Design review of the part shown in the three views and the two pictorial views. Dimensions are in mm from the part's minimum x, y and z. A direction names the side the tool comes from. Give positions to 0.01 mm unless a question says otherwise; leave off trailing zeros. Order: outer loops, then holes, each group sorted by start corner. A loop starts at its lowest first (then second) coordinate and runs counter-clockwise, first axis right, second up.
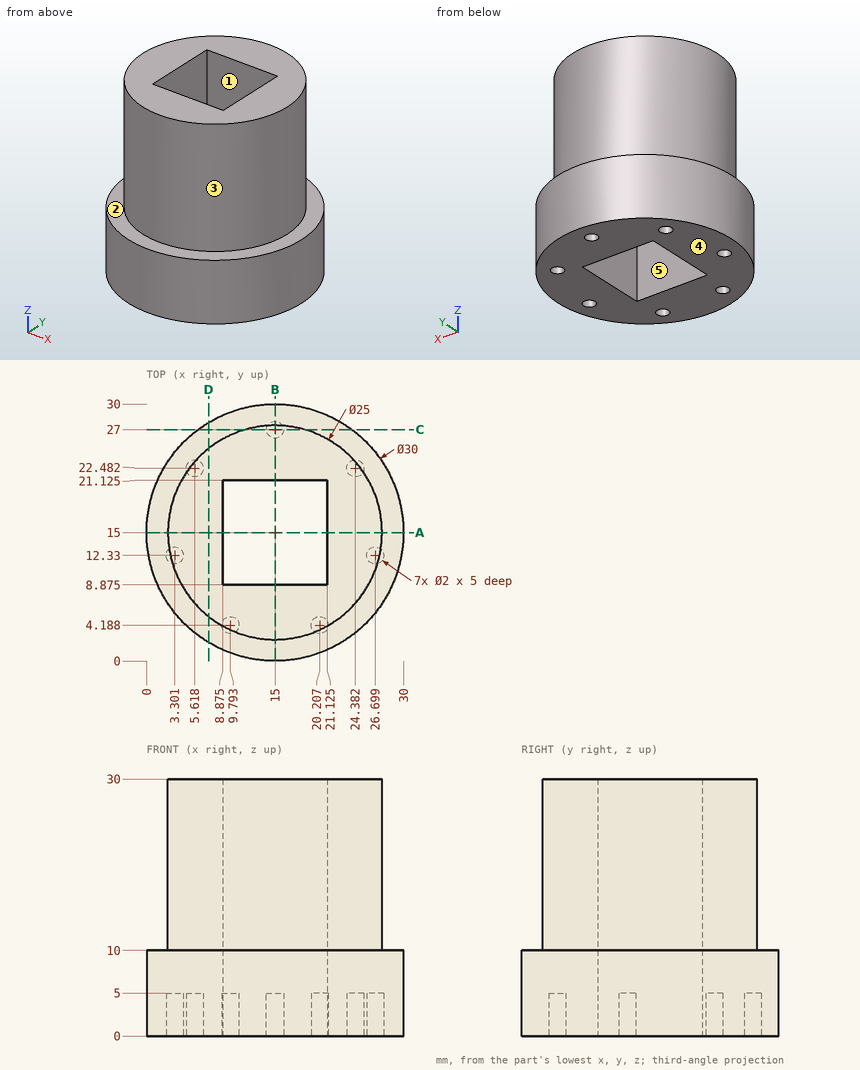
1) Tool access review of the marked faces 4 and 5: name each direction out of +Z, -Z, +X, -X, +Y, -Y from which nothing blocks a thin tool from reaching the whole face with its end or side.
Answer sheet:
face 4: -Z, +X, -X, +Y, -Y
face 5: +Z, -Z
2) Draft analysis for pull direction X (two halves, no side actions). For the marked faces 1, 2 and 3, state which applies: +X half, -X half, draft (parallel to the pull), parting line (faces both ways), or undercut.
Answer sheet:
face 1: undercut
face 2: draft
face 3: parting line
3) We need section B-B on x = 15. Give the boundary of the cut face in (y, z) (1 decimal).
Answer sheet:
outline: (0, 0) - (8.9, 0) - (8.9, 30) - (2.5, 30) - (2.5, 10) - (0, 10) - close; (21.1, 0) - (26, 0) - (26, 5) - (28, 5) - (28, 0) - (30, 0) - (30, 10) - (27.5, 10) - (27.5, 30) - (21.1, 30) - close
4) We need section A-A on y = 15. Give the boundary of the cut face in (x, z) (1 decimal).
Answer sheet:
outline: (0, 0) - (8.9, 0) - (8.9, 30) - (2.5, 30) - (2.5, 10) - (0, 10) - close; (21.1, 0) - (30, 0) - (30, 10) - (27.5, 10) - (27.5, 30) - (21.1, 30) - close
5) We need section C-C on y = 27. Give the boundary of the cut face in (x, z).
Answer sheet:
outline: (6, 0) - (14, 0) - (14, 5) - (16, 5) - (16, 0) - (24, 0) - (24, 10) - (18.5, 10) - (18.5, 30) - (11.5, 30) - (11.5, 10) - (6, 10) - close
6) To check wall thickness, follow line 1 (X direction, y = 22.75, z = 3) (1 decimal); line 2 (Z direction, x = 8.5, y = 27.5); line 3 (X direction, y = 20, z = 26.75) (1 decimal). State the ranges of each line that lie inside material, in increasing order.
Answer sheet:
line 1: x = 2.2 to 4.7, 6.6 to 23.4, 25.3 to 27.8
line 2: z = 0 to 10
line 3: x = 3.5 to 8.9, 21.1 to 26.5
7) Clearance check with flat-ended pins moving along their axes: pin 1 (0.6 mm diameter, centred on x = 5.5, y = 22.5, fed in from -Z); pin 2 (3.5 mm diameter, centred on x = 14.5, z = 18.5, fed in from -Y); pin 3 (8 mm diameter, centred on x = 10.5, z = 6.5, fed in from -Y). State where each tip first meets the part, or that it passes through.
Answer sheet:
pin 1: stops at z = 5
pin 2: stops at y = 2.5
pin 3: stops at y = 0.01
8) We need section D-D on x = 7.25. Give the boundary of the cut face in (y, z).
Answer sheet:
outline: (2.16, 0) - (27.84, 0) - (27.84, 10) - (24.81, 10) - (24.81, 30) - (5.19, 30) - (5.19, 10) - (2.16, 10) - close
